from build123d import *

# Parameters (mm, degrees)
F0_W      = 37.25
F0_H      = 49.5
F1_DEPTH  = 27
F2_W      = 29.25
F2_H      = 23
F3_DEPTH  = 49.501
F4_W      = 2.3
F4_H      = 3
F5_DEPTH  = 49.501
F6_R      = 5
F7_R      = 3.125
F8_DEPTH  = 20
F10_DEPTH = 27.001
F12_DEPTH = 23
F13_W     = 33.85
F13_H     = 3
F14_DEPTH = 12.982547
F15_R     = 1.125
F16_DEPTH = 20


with BuildPart() as f1:
    # F0 (on Top) → F1 (new body)
    with BuildSketch(Plane.XY):
        Rectangle(F0_W, F0_H)
    extrude(amount=F1_DEPTH)

    # F2 (on face) → F3 (cut, through all)
    with BuildSketch(Plane.XZ.offset(24.75)):
        with Locations((0, 15.5)):
            Rectangle(F2_W, F2_H)
    extrude(amount=-F3_DEPTH, mode=Mode.SUBTRACT)

    # F4 (on face) → F5 (cut, through all)
    with BuildSketch(Plane.XZ.offset(24.75)):
        with Locations((-15.775, 25.5)):
            Rectangle(F4_W, F4_H)
        with Locations((15.775, 25.5)):
            Rectangle(F4_W, F4_H)
    extrude(amount=-F5_DEPTH, mode=Mode.SUBTRACT)

    # F6
    f6_edges = [f1.edges().sort_by_distance(p)[0] for p in [
        (18.625, 0, 0),
        (-18.625, 0, 0),
    ]]
    fillet(f6_edges, radius=F6_R)

    # F7 (on face) → F8 (join, through all)
    with BuildSketch(Plane.XY.offset(4)):
        with Locations((0, 15.75)):
            Circle(F7_R)
    extrude(amount=F8_DEPTH)

    # F9 (on face) → F10 (cut, through all)
    with BuildSketch(Plane(origin=(0, 0, 0), x_dir=(1, 0, 0), z_dir=(0, 0, -1))):
        with BuildLine():
            Line((-18.625, -24.75), (18.625, -24.75))
            ThreePointArc((18.625, -24.75), (0, -22.75), (-18.625, -24.75))
        make_face()
    extrude(amount=-F10_DEPTH, mode=Mode.SUBTRACT)

    # F11 (on face) → F12 (join, through all)
    with BuildSketch(Plane.XY.offset(4)):
        Polygon((17.763313, 14.75), (0, 14.75), (-17.661568, 14.75), (-17.661568, 11.768454), (17.763313, 11.768454), align=None)
    extrude(amount=F12_DEPTH)

    # F13 (on face) → F14 (cut, through all)
    with BuildSketch(Plane.XZ.offset(-11.768454)):
        with Locations((0, 25.5)):
            Rectangle(F13_W, F13_H)
    extrude(amount=-F14_DEPTH, mode=Mode.SUBTRACT)

    # F15 (on face) → F16 (cut, through all)
    with BuildSketch(Plane.XY.offset(24)):
        with Locations((0, 15.75)):
            Circle(F15_R)
    extrude(amount=-F16_DEPTH, mode=Mode.SUBTRACT)


solid = f1.part
Verification items for the finished model (mm, model axes). A direction names the side the tool comes from. Round coordinates to 2 decimals unless told otherwise and drop trailing zeros. Loops run counter-clockwise (first coordinate to the right, second up) from the corner with the lowest first, then second, coordinate; pieces in that order, holes last. Notation, with made-up numbers: (-1.75, 0.5) - (30.25, 0.5) arc R18 ccw to (30.25, 32.5) - close; hole circle Ø3 at (-37.75, 82.5). An arc over 180 degrees is marked (long way). Answer in a Markdown table with one row per item. Add a question column.
Q1. Section check D-D on y = 2. Enter the section's corners in (x, z) (3 decimals).
Q2. Release check for a two-part mould opening along X. For faces 6 (the face through (0, -24.75, 3)), 7 (the face through (0.09, 22.75, 3.44)), 8 (the face through (18.625, 0, 16)), 9 (the face through (-14.625, -7, 14)) record: pulls with the +X half, pulls with the -X half, needs draft (parallel to the pull), parting line crosses it, or undercut.
Q3. Section check C-C on x = 0. Enter the section's corners in (y, z) (3 decimals).
Q4. Section check A-A on z = 21.5. Enter the section's corners in (x, y) (3 decimals), plus the area to 3 significant figures.
Q5. Gauge pin test, flat ends, axial feed: pin 1 (10 mm diameter, centred on x = -2.5, y = 8.5, fed in from +Z); pin 2 (10 mm diameter, centred on x = -5.5, z = 15, fed in from -Y); pin 3 (9 mm diameter, centred on x = -1.5, y = 1.5, fed in from +Z). Record the tip position at first contact, or that the pin passes through.
Q6. Material ranges on line 1 (X direction, y = 21.5, z = 18) (3 decimals); line 2 (Y direction, x = 0, z = 14.75) (3 decimals); line 3 (Z direction, x = 6.5, y = 20.5), recorded low to high.
Q7. Tool access check on faces 1 (the face through (-16.925, -1, 25)), 2 (the face through (0, 16, 4)), 3 (the face through (-18.625, 0, 16)), 4 (the face through (14.625, -7, 14)), 5 (the face through (14.625, 19, 14)). Record the directions out of +Z, -Z, +X, -X, +Y, -Y that give a thin tool (end or side, any length) a straight path to the whole face; none if there is none.
Q8. Section check B-B on y = 13. Enter the section's corners in (x, z) (3 decimals).
Found:
| question | item | result |
|---|---|---|
| 1 | outline | (-18.625, 5) arc R5 ccw to (-13.625, 0) - (13.625, 0) arc R5 ccw to (18.625, 5) - (18.625, 27) - (16.925, 27) - (16.925, 24) - (14.625, 24) - (14.625, 4) - (-14.625, 4) - (-14.625, 24) - (-16.925, 24) - (-16.925, 27) - (-18.625, 27) - close |
| 2 | face 6 | needs draft |
| 2 | face 7 | undercut |
| 2 | face 8 | pulls with the +X half |
| 2 | face 9 | undercut |
| 3 | outline | (-24.75, 0) - (22.75, 0) - (22.75, 4) - (18.875, 4) - (18.875, 24) - (16.875, 24) - (16.875, 4) - (14.625, 4) - (14.625, 24) - (11.768, 24) - (11.768, 4) - (-24.75, 4) - close |
| 4 | outline | (-18.625, -24.75) - (-14.625, -24.75) - (-14.625, 11.768) - (14.625, 11.768) - (14.625, -24.75) - (18.625, -24.75) - (18.625, 24.75) arc R87.723 cw to (14.625, 23.978) - (14.625, 14.75) - (2.961, 14.75) arc R3.125 ccw (long way) to (-2.961, 14.75) - (-14.625, 14.75) - (-14.625, 23.978) arc R87.723 cw to (-18.625, 24.75) - close; hole circle Ø2.25 at (0, 15.75) |
| 4 | area | 497 mm² |
| 5 | pin 1 | stops at z = 24 |
| 5 | pin 2 | stops at y = 11.77 |
| 5 | pin 3 | stops at z = 4 |
| 6 | line 1 | x = -18.625 to -14.625, 14.625 to 18.625 |
| 6 | line 2 | y = 11.768 to 14.625, 16.875 to 18.875 |
| 6 | line 3 | z = 0 to 4 |
| 7 | face 1 | +Z, +Y, -Y |
| 7 | face 2 | +Z |
| 7 | face 3 | +Z, -Z, -X, +Y, -Y |
| 7 | face 4 | +Z, -Y |
| 7 | face 5 | +Z, +Y |
| 8 | outline | (-18.625, 5) arc R5 ccw to (-13.625, 0) - (13.625, 0) arc R5 ccw to (18.625, 5) - (18.625, 27) - (16.925, 27) - (16.925, 24) - (-16.925, 24) - (-16.925, 27) - (-18.625, 27) - close |
